Input: dimensioned drawing with shaded views. Units: mm. Origin: part minimum x, y, z. A direction names the side the tool comes from. Round coordinates to 2 decimals unless told otherwise and drop trailing zeros. Order: outer loops, then holes, each group sorted by start corner. A loop starts at its lowest first (then second) coordinate and runs counter-clockwise, first axis right, second up.
Item 1: First-contact query: pin 1 (1.3 mm diameter, centred on x = 1.5, z = 8.5, fed in from -Y); pin 2 (5 mm diameter, centred on y = 19, z = 8, fed in from +X); pin 3 (1.5 mm diameter, centred on y = 48, z = 9.5, fed in from -X). Flat tips, straight axial feed; report the tip coordinate or a pass-through.
Item 2: Cut plane D-D on y = 22.5. Output: boundary loops of the cut face in (x, z), then the cut area to 3 significant figures.
Item 3: Cut plane B-B on z = 6.35. Output: boundary loops of the cut face in (x, y), then the cut area to 3 significant figures.
Item 4: Line query: L1, parallel to X at y = 4, z = 11.25; L2, parallel to Z at x = 6.25, y = 6.35; L3, parallel to Z at x = 7.5, y = 6.35 (1 decimal). Output: solid intervals per line, ascending.
Item 5: Reachability of the marked faces 1, 2 and 3 from +Z, -Z, +X, -X, +Y, -Y: full face, straight path, thin tool, end or side. Return the list, or none.
Item 6: Cut plane A-A on y = 6.35. Output: boundary loops of the cut face in (x, z), then the cut area to 3 significant figures.
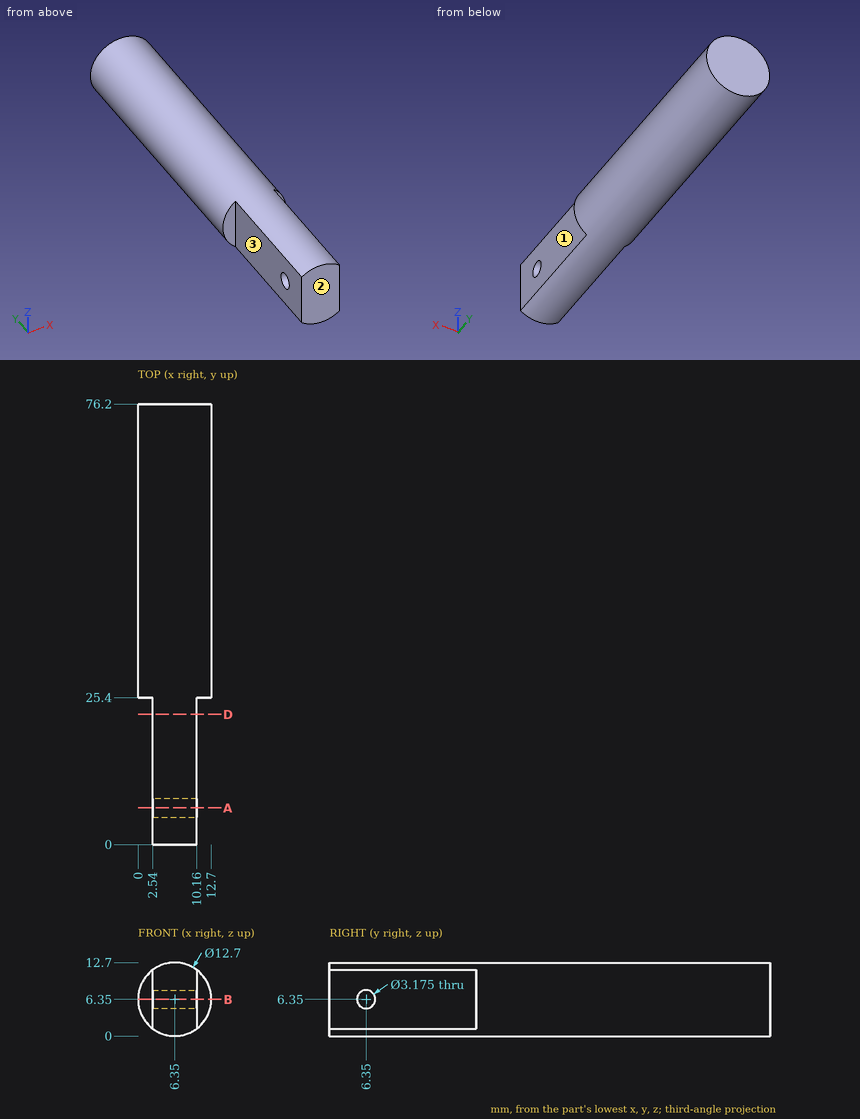
From the geometry:
1. pin 1: stops at y = 25.4
1. pin 2: stops at x = 10.16
1. pin 3: stops at x = 0.47
2. outline: (2.54, 1.27) arc R6.35 ccw to (10.16, 1.27) - (10.16, 11.43) arc R6.35 ccw to (2.54, 11.43) - close
2. area: 90.6 mm2
3. outline: (0, 25.4) - (2.54, 25.4) - (2.54, 7.94) - (10.16, 7.94) - (10.16, 25.4) - (12.7, 25.4) - (12.7, 76.2) - (0, 76.2) - close; (2.54, 0) - (10.16, 0) - (10.16, 4.76) - (2.54, 4.76) - close
3. area: 815 mm2
4. L1: x = 2.54 to 10.16
4. L2: z = 0 to 4.76, 7.94 to 12.7
4. L3: z = 0.1 to 4.8, 7.9 to 12.6
5. face 1: +Z, -Z, +X, -Y
5. face 2: +Z, -Z, +X, -X, -Y
5. face 3: +Z, -Z, -X, -Y
6. outline: (2.54, 1.27) arc R6.35 ccw to (10.16, 1.27) - (10.16, 4.76) - (2.54, 4.76) - close; (2.54, 7.94) - (10.16, 7.94) - (10.16, 11.43) arc R6.35 ccw to (2.54, 11.43) - close
6. area: 66.4 mm2
